The listing builds one solid part. Answer for the finished solid, in the listing's coordinates (mm). Face numbers are marked on the shaded views. A direction names the side the tool comes from. Coordinates: 2 decimals unless noted, no trailing zeros. Loops run counter-clockwise (first coordinate to the right, second up) from the corner with the lowest first, then second, coordinate; pieces in that order, holes last. Notation, with made-up numbers: (79.25, 69.25) - (93.25, 69.25) arc R15 ccw to (93.25, 86.25) - close; hole circle Ø3 at (31.5, -3.5). An arc over 180 degrees is marked (long way). Put each result on its own line as item: value.
```python
from build123d import *

# Parameters (mm, degrees)
F1_DEPTH = 25.4
F2_W     = 8.498132
F2_H     = 12.7
F3_DEPTH = 12.7


with BuildPart() as f1:
    # F0 (on Right) → F1 (new body)
    with BuildSketch(Plane.YZ):
        Polygon((0, 0), (25.4, 0), (25.4, 31.75), (12.7, 31.75), (12.7, 6.35), (0, 6.35), align=None)
    extrude(amount=F1_DEPTH)

    # F2 (on face) → F3 (cut, symmetric)
    with BuildSketch(Plane.XY.offset(31.75)):
        with Locations((12.980955, 19.05)):
            Rectangle(F2_W, F2_H)
    extrude(amount=F3_DEPTH, both=True, mode=Mode.SUBTRACT)


solid = f1.part
```
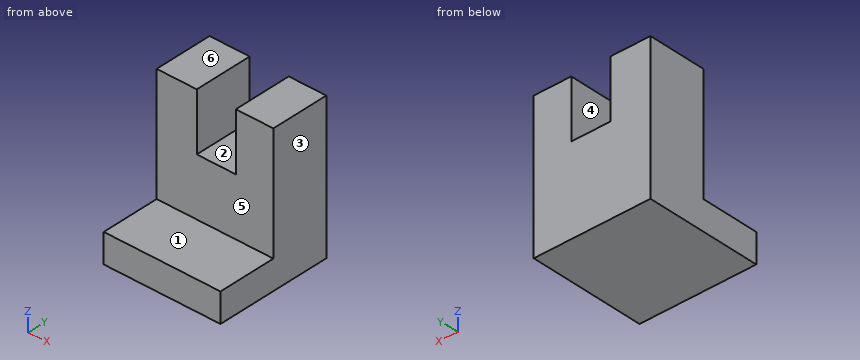
1) Straight lines are drawn through the part: L1, parallel to X at y = 15, z = 19.5; L2, parallel to Y at x = 3.5, z = 19; L3, parallel to Z at x = 9.75, y = 16.25. For each, find the intervals that lie inside material, in ascending order. Write a range as [from, to].
Found:
L1: x = [0, 8.73], [17.23, 25.4]
L2: y = [12.7, 25.4]
L3: z = [0, 19.05]
2) Each of these flat-tipped pins is pushed along its axis until it touches: pin 1 (3 mm diameter, centred on x = 10, y = 9, fed in from +Z); pin 2 (4 mm diameter, centred on x = 12, y = 16, fed in from +Z); pin 3 (10 mm diameter, centred on x = 11.5, y = 21, fed in from -Z). Where does it stop, or does it pass through?
Found:
pin 1: stops at z = 6.35
pin 2: stops at z = 19.05
pin 3: stops at z = 0
3) The part is cut by section B-B (y = 19). Give the vertices of the cut face in (x, z), and give its area (3 significant figures).
Found:
outline: (0, 0) - (25.4, 0) - (25.4, 31.75) - (17.23, 31.75) - (17.23, 19.05) - (8.73, 19.05) - (8.73, 31.75) - (0, 31.75) - close
area: 699 mm^2
4) For a pull along X with two mould halves and no side action, classify the marked faces 1, 2 and 3 as pulls with the +X half, pulls with the -X half, needs draft (parallel to the pull), parting line crosses it, or undercut.
Found:
face 1: needs draft
face 2: undercut
face 3: pulls with the +X half
5) For the marked faces 4, 5 and 6, determine the directions among +Z, -Z, +X, -X, +Y, -Y from which every point of the face is accessible in a straight line to the end or side of a thin tool.
Found:
face 4: +Z, +Y, -Y
face 5: +Z, +X, -X, -Y
face 6: +Z, +X, -X, +Y, -Y
6) The part is cut by section A-A (x = 16). Give the vertices of the cut face in (y, z), and give its area (3 significant figures).
Found:
outline: (0, 0) - (25.4, 0) - (25.4, 19.05) - (12.7, 19.05) - (12.7, 6.35) - (0, 6.35) - close
area: 323 mm^2
7) The part is cut by section C-C (z = 12). Give the vertices of the cut face in (x, y), and give its area (3 significant figures).
Found:
outline: (0, 12.7) - (25.4, 12.7) - (25.4, 25.4) - (0, 25.4) - close
area: 323 mm^2
8) The part is cut by section D-D (x = 2.5). Give the vertices of the cut face in (y, z).
Found:
outline: (0, 0) - (25.4, 0) - (25.4, 31.75) - (12.7, 31.75) - (12.7, 6.35) - (0, 6.35) - close
